Geometry: final body of the model. Coordinates: model frame, mm. A direction names the side the tool comes from. Round coordinates to 2 decimals unless told otherwise and drop trailing zeros. Loops run counter-clockwise (first coordinate to the right, second up) from the corner with the lowest first, then second, coordinate; pieces in that order, holes last. Notation, with made-up numbers: (85.25, -21) - (139.25, -21) arc R17 cw to (139.25, -8) - close; hole circle Ø1 at (55.5, 71.25). An arc over 180 degrees is marked (long way). Answer as CSV lines item,"result".
from build123d import *

# Parameters (mm, degrees)
SKETCH1_W           = 90
SKETCH1_H           = 60
BOSS_EXTRUDE1_DEPTH = 4
SKETCH2_R           = 1.7
SKETCH2_R_2         = 2.15
CUT_EXTRUDE1_DEPTH  = 4
CUT_EXTRUDE2_DEPTH  = 2
BOSS_EXTRUDE2_DEPTH = 4
SKETCH5_R           = 9.5
CUT_EXTRUDE3_DEPTH  = 2
FILLET3_R           = 5
FILLET4_R           = 5


with BuildPart() as part:
    # Sketch1 → Boss-Extrude1 (new body)
    with BuildSketch(Plane(origin=(0, 0, 0), x_dir=(1, 0, 0), z_dir=(0, 1, 0))):
        Rectangle(SKETCH1_W, SKETCH1_H)
    extrude(amount=BOSS_EXTRUDE1_DEPTH)

    # Sketch2 → Cut-Extrude1 (cut)
    with BuildSketch(Plane(origin=(0, 4, 0), x_dir=(1, 0, 0), z_dir=(0, 1, 0))):
        with Locations(Location((-39, 24, 0), (0, 0, 270))):
            Circle(SKETCH2_R)
        with Locations(Location((-39, -24, 0), (0, 0, 270))):
            Circle(SKETCH2_R)
        with Locations(Location((39, -24, 0), (0, 0, 270))):
            Circle(SKETCH2_R)
        with Locations(Location((39, 24, 0), (0, 0, 270))):
            Circle(SKETCH2_R)
        with Locations(Location((-34.4, 0, 0), (0, 0, 270))):
            Circle(SKETCH2_R_2)
        with Locations(Location((34.4, 0, 0), (0, 0, 270))):
            Circle(SKETCH2_R_2)
    extrude(amount=-CUT_EXTRUDE1_DEPTH, mode=Mode.SUBTRACT)

    # Sketch3 → Cut-Extrude2 (cut)
    with BuildSketch(Plane.XZ):
        Polygon((-30.825, 2.064027212), (-34.4, 4.128054425), (-37.975, 2.064027212), (-37.975, -2.064027212), (-34.4, -4.128054425), (-30.825, -2.064027212), align=None)
        Polygon((37.975, 2.064027212), (34.4, 4.128054425), (30.825, 2.064027212), (30.825, -2.064027212), (34.4, -4.128054425), (37.975, -2.064027212), align=None)
    extrude(amount=-CUT_EXTRUDE2_DEPTH, mode=Mode.SUBTRACT)

    # Sketch4 → Boss-Extrude2 (add)
    with BuildSketch(Plane(origin=(0, 4, 0), x_dir=(1, 0, 0), z_dir=(0, 1, 0))):
        with BuildLine():
            Line((-45, 22), (-45, -22))
            ThreePointArc((-45, -22), (-67, 0), (-45, 22))
        make_face()
    extrude(amount=-BOSS_EXTRUDE2_DEPTH)

    # Sketch5 → Cut-Extrude3 (cut)
    with BuildSketch(Plane(origin=(0, 4, 0), x_dir=(1, 0, 0), z_dir=(0, 1, 0))):
        with Locations(Location((-54.5, 0, 0), (0, 0, 270))):
            Circle(SKETCH5_R)
    extrude(amount=-CUT_EXTRUDE3_DEPTH, mode=Mode.SUBTRACT)

    # Fillet3
    fillet3_edges = [part.edges().sort_by_distance(p)[0] for p in [
        (-45, 2, -30),
        (45, 2, -30),
        (45, 2, 30),
        (-45, 2, 30),
    ]]
    fillet(fillet3_edges, radius=FILLET3_R)

    # Fillet4
    fillet4_edges = [part.edges().sort_by_distance(p)[0] for p in [
        (-45, 2, -22),
        (-45, 2, 22),
    ]]
    fillet(fillet4_edges, radius=FILLET4_R)


solid = part.part
(1) Section B-B (y = 2.95). Give the number of separate pieces and of enclosed holes in the cut face, and give its area (3 significant figures).
Findings below:
separate pieces,"1"
enclosed holes,"7"
area,"5,800 mm2"
(2) Pin query (flat end, axial travel): P1, Ø17, axis at x = -54.5, z = 0, coming from the +Y side; P2, Ø2, axis at x = -45.5, y = 0.5, coming from the +Z side; P3, Ø1, axis at y = 1, z = 0, coming from the -X side. Return the tip coordinate at first contact, or that it passes through.
Findings below:
P1,"y = 2"
P2,"z = 27.18"
P3,"x = -67"
(3) Draft query along X for faces 1 (the face through (-12, 0, 0)), 2 (the face through (-67, 2, 0)), 3 (the face through (37.5, 2, -23.2)). Return one class per face: pulls with the +X half, pulls with the -X half, needs draft (parallel to the pull), parting line crosses it, or undercut.
Findings below:
face 1,"needs draft"
face 2,"pulls with the -X half"
face 3,"undercut"
(4) Access query for faces 4 (the face through (-36.16, 0.99, 3.11)), 5 (the face through (37.5, 2, 24.8)), 6 (the face through (-63.774, 3.014, -2.059)). Directions: +Z, -Z, +X, -X, +Y, -Y. A direction counts if a zero-diameter tool reaches every point of the face in a straight line with its end or side. Return the directions, or none.
Findings below:
face 4,"-Y"
face 5,"+Y, -Y"
face 6,"+Y"
(5) Section A-A (z = 0). Output: boundary loops of the cut face in (x, y) (3 decimals).
Findings below:
outline,"(-67, 0) - (-37.975, 0) - (-37.975, 2) - (-36.55, 2) - (-36.55, 4) - (-45, 4) - (-45, 2) - (-64, 2) - (-64, 4) - (-67, 4) - close; (-32.25, 2) - (-30.825, 2) - (-30.825, 0) - (30.825, 0) - (30.825, 2) - (32.25, 2) - (32.25, 4) - (-32.25, 4) - close; (36.55, 2) - (37.975, 2) - (37.975, 0) - (45, 0) - (45, 4) - (36.55, 4) - close"
(6) Material intervals for line 1 along X through (y, z) = (2.55, 0); line 2 along X through (y, z) = (0.3, -25.5); line 3 along X through (y, z) = (1.25, 24), sorted ascending.
Findings below:
line 1,"-67 to -64, -45 to -36.55, -32.25 to 32.25, 36.55 to 45"
line 2,"-44.99 to -39.8, -38.2 to 38.2, 39.8 to 44.97"
line 3,"-45.58 to -40.7, -37.3 to 37.3, 40.7 to 45"
(7) Section C-C (z = 16). Output: boundary loops of the cut face in (x, y), and give its area (3 significant figures).
Findings below:
outline,"(-60.1, 0) - (45, 0) - (45, 4) - (-60.1, 4) - close"
area,"420 mm2"
